Verification items for this drawing (mm, ordinates from the low corner). Coordinates: 2 decimals unless noted, no trailing zeros. Order: outer loops, then holes, each group sorted by start corner. A loop starts at its lowest first (then second) coordinate and runs counter-clockwise, first axis right, second up. Notation, with made-up numbers: M 28.5,40 L 62.5,40 A17 cw 62.5,61 Z; hole C 28,19 d11. An arc over 180 degrees is marked long. Answer as a JSON object with one key per item and string values. Group by question number.
(1) Cross-section at B-B (x = 50). Enter the section's corners in (y, z) (3 decimals).
(2) Material ranges on line 1 (Z direction, x = 50, y = 3.55) (3 decimals); line 2 (X direction, y = 2.65, z = 25) (1 decimal); line 3 (Z direction, x = 56, y = 2.15), recorded low to high.
(3) Gauge pin test, flat end, axial feed: pin 1 Ø3 at (x, y) = (39.5, 1) entering from -Z. Record the tip position at first contact, or that the pin passes through.
(4) Cross-section at A-A (z = 25). Enter the section's corners in (x, y) (1 decimal).
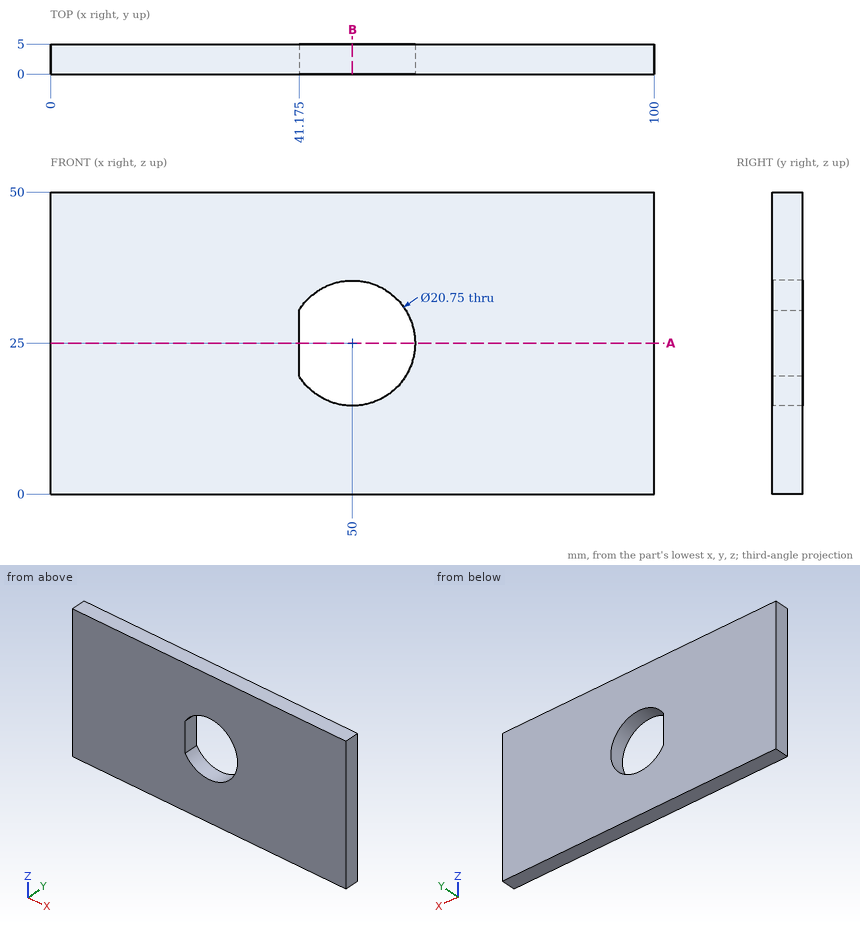
Taken from the geometry:
{
 "1": {"outline": "M 0,0 L 5,0 L 5,14.625 L 0,14.625 Z; M 0,35.375 L 5,35.375 L 5,50 L 0,50 Z"},
 "2": {"line 1": "z = 0 to 14.625, 35.375 to 50", "line 2": "x = 0 to 41.2, 60.4 to 100", "line 3": "z = 0 to 16.54, 33.46 to 50"},
 "3": {"pin 1": "stops at z = 0"},
 "4": {"outline": "M 0,0 L 41.2,0 L 41.2,5 L 0,5 Z; M 60.4,0 L 100,0 L 100,5 L 60.4,5 Z"}
}
